```python
from build123d import *

# Parameters (mm, degrees)
BOSS_EXTRUDE2_DEPTH = 30
FILLET1_R           = 20
SKETCH7_R           = 1.5
CUT_EXTRUDE2_DEPTH  = 79.379142634


with BuildPart() as part:
    # Sketch6 → Boss-Extrude2 (new body)
    with BuildSketch(Plane(origin=(0, 0, 0), x_dir=(0, 0, -1), z_dir=(1, 0, 0))):
        Polygon((0, 0), (10, 0), (10, 34.8), (53.5, 34.8), (53.5, 0), (63.5, 0), (63.5, -3), (50.5, -3), (50.5, 31.8), (13, 31.8), (13, -3), (0, -3), align=None)
    extrude(amount=BOSS_EXTRUDE2_DEPTH)

    # Fillet1
    # the kernel refuses this fillet: 20 mm, written as the material it adds along each edge
    with BuildSketch(Plane(origin=(0, 31.8, -13), x_dir=(0, 0, -1), z_dir=(1, 0, 0)), Plane(origin=(0, 31.8, -50.5), x_dir=(0, -1, 0), z_dir=(1, 0, 0))) as fillet1_piece_1:
        with BuildLine():
            CenterArc((FILLET1_R, -FILLET1_R), FILLET1_R, 90, 90)
            Line((0, -FILLET1_R), (0, 0))
            Line((0, 0), (FILLET1_R, 0))
        make_face()
    extrude(amount=30)
    # the kernel refuses this fillet: 20 mm, written as the material it takes off along each edge
    with BuildSketch(Plane(origin=(-50, 34.8, -10), x_dir=(0, -1, 0), z_dir=(1, 0, 0)), Plane(origin=(-50, 34.8, -53.5), x_dir=(0, 0, 1), z_dir=(1, 0, 0))) as fillet1_2_piece_1:
        with BuildLine():
            CenterArc((FILLET1_R, FILLET1_R), FILLET1_R, 180, 90)
            Line((0, FILLET1_R), (0, 0))
            Line((0, 0), (FILLET1_R, 0))
        make_face()
    extrude(amount=130, mode=Mode.SUBTRACT)

    # Sketch7 → Cut-Extrude2 (cut, through all)
    with BuildSketch(Plane(origin=(0, 0, 0), x_dir=(1, 0, 0), z_dir=(0, 1, 0))):
        with Locations(Location((27, 60.5, 0), (0, 0, 270))):
            Circle(SKETCH7_R)
        with Locations(Location((3, 60.5, 0), (0, 0, 270))):
            Circle(SKETCH7_R)
        with Locations(Location((3, 3, 0), (0, 0, 270))):
            Circle(SKETCH7_R)
        with Locations(Location((27, 3, 0), (0, 0, 270))):
            Circle(SKETCH7_R)
    extrude(amount=-CUT_EXTRUDE2_DEPTH, mode=Mode.SUBTRACT)


solid = part.part
```
CAD build for the part. Positions are in the model's coordinates, mm. A direction names the side the tool comes from. Coordinates: 2 decimals unless noted, no trailing zeros. Loops run counter-clockwise (first coordinate to the right, second up) from the corner with the lowest first, then second, coordinate; pieces in that order, holes last. Notation, with made-up numbers: (60, -6) - (72, -6) arc R33 cw to (72, 25) - close; hole circle Ø9 at (62.5, 20). An arc over 180 degrees is marked (long way). Use CSV: the item, a comma, the result in double quotes. Start each with the question number.
Q1. Cut at C-C, the plane y = 6. List the corners of the cut face in (x, z).
Q2. 3-axis set-ups, long thin cutter, end or side, ignore diameter. For faces 4 (the flat face through (15, 4, -50.5)), 5 (the flat face through (15, 34.8, -32)), 6 (the flat face through (15, 0, -5)): which of +Z, -Z, +X, -X, +Y, -Y reach the whole face in a straight line?
Q3. Cut at B-B, the plane z = -60.5. List the corners of the cut face in (x, y), then the cut area to 3 significant figures.
Q4. Drop flat-ended pins along their axis: P1, Ø4, axis at x = 3, z = -60.5, coming from the -Y side; P2, Ø5, axis at x = 17, z = -57, coming from the +Y side; P3, Ø3, axis at x = 21, z = -38.5, coming from the -Y side; P4, Ø8, axis at x = 10.5, y = 23, coming from the +Z side. Give the stop position or say it passes through.
Q5. Probe probe 1 along X at (y, z) = (-1.55, -60.5); probe 2 along X at (y, z) = (-2, -60); probe 3 along Z at (x, y) = (6.5, 29). List the from-to ranges inside material, lowest first. Write a range as from..to.
Q6. Two-plate mould, pull along X, no slides. Class faces 1 (the flat face through (15, 0, -58)), 2 (the flat face through (30, 22, -48)), 3 (the cylindrical face through (28.265, -1.479, -59.694)): +X half, -X half, draft (parallel to the pull), parting line (faces both ways), or undercut.
Q7. Cut at D-D, the plane y = 30.5. List the corners of the cut face in (x, z), then the cut area to 3 significant figures.
Q8. Cut at A-A, the plane x = 3. List the corners of the cut face in (y, z), then the cut area to 3 significant figures.
Here are the results:
1,outline,"(0, -53.5) - (30, -53.5) - (30, -50.5) - (0, -50.5) - close; (0, -13) - (30, -13) - (30, -10) - (0, -10) - close"
2,face 4,"+X, -X, -Y"
2,face 5,"+Z, -Z, +X, -X, +Y"
2,face 6,"+Z, +X, -X, +Y"
3,outline,"(0, -3) - (1.5, -3) - (1.5, 0) - (0, 0) - close; (4.5, -3) - (25.5, -3) - (25.5, 0) - (4.5, 0) - close; (28.5, -3) - (30, -3) - (30, 0) - (28.5, 0) - close"
3,area,"72.0 mm2"
4,P1,"y = -3"
4,P2,"y = 0"
4,P3,"y = 29.4"
4,P4,"z = -10.45"
5,probe 1,"0..1.5, 4.5..25.5, 28.5..30"
5,probe 2,"0..1.59, 4.41..25.59, 28.41..30"
5,probe 3,"-47.58..-40.71, -22.79..-15.92"
6,face 1,"draft"
6,face 2,"+X half"
6,face 3,"undercut"
7,outline,"(0, -45.89) - (30, -45.89) - (30, -37.59) - (0, -37.59) - close; (0, -25.91) - (30, -25.91) - (30, -17.61) - (0, -17.61) - close"
7,area,"498 mm2"
8,outline,"(-3, -63.5) - (0, -63.5) - (0, -62) - (-3, -62) - close; (-3, -59) - (0, -59) - (0, -53.5) - (14.8, -53.5) arc R20 ccw to (34.8, -33.5) - (34.8, -30) arc R20 ccw to (14.8, -10) - (0, -10) - (0, -4.5) - (-3, -4.5) - (-3, -13) - (11.8, -13) arc R20 cw to (31.76, -31.75) arc R20 cw to (11.8, -50.5) - (-3, -50.5) - close; (-3, -1.5) - (0, -1.5) - (0, 0) - (-3, 0) - close"
8,area,"381 mm2"
